Autodesk Inventor part; units mm, degrees
ref_plane "YZ Plane" through (0, 0, 0) normal (1, 0, 0) x (0, 1, 0)
ref_plane "XZ Plane" through (0, 0, 0) normal (0, 1, 0) x (-1, 0, 0)
ref_plane "XY Plane" through (0, 0, 0) normal (0, 0, 1) x (1, 0, 0)
sketch "Sketch1" plane through (0, 0, 0) normal (1, 0, 0) x (0, 1, 0)
  circle A0 centre (-9.1612, 46.1081) radius 0.5 construction
  circle A1 centre (-9.1612, 46.1081) radius 0.9 construction
  line L0 (0, 43.0329) -> (-28.9151, 45.5627) construction
  line L1 (1.0918, 43.1767) -> (-27.4928, 38.1364) construction
  line L2 (-1.0918, 51.3262) -> (-28.367, 41.3989) construction
  line L3 (0, 51.4699) -> (-28.9151, 48.9402) construction
  line L4 (17.609, 51.9698) -> (-38.9081, 36.826) construction
  line L5 (18.2302, 47.2514) -> (-40.2807, 47.2514) construction
  line L6 (-2.4562, 42.2517) -> (-3.9425, 12.3724) construction
  line L7 (-19.1091, 33.3894) -> (19.1091, 33.3894) construction
  line L8 (-15.9499, 49.3393) -> (15.9499, 17.4395) construction
  line L9 (-15.9953, 17.3941) -> (15.9953, 49.3847) construction
  line L10 (2.4672, 42.2517) -> (3.9506, 12.3724) construction
  line L11 (-4.2099, 47.2514) -> (-6.25, 6.2414) construction
  line L12 (4.2215, 47.2514) -> (6.2448, 6.4952) construction
  circle A2 centre (-12.7187, 42.5506) radius 0.9 construction
  line L13 (-11.8457, 45.2351) -> (-10.9619, 46.119) construction
  line L14 (-10.9619, 46.119) -> (-9.1941, 44.3513) construction
  line L15 (-12.7296, 44.3513) -> (-13.501, 42.9956) construction
  line L16 (-11.8457, 45.2351) -> (-12.7296, 44.3513) construction
  line L17 (-10.9619, 42.5835) -> (-12.2433, 41.7864) construction
  line L18 (-12.7296, 44.3513) -> (-10.9619, 42.5835) construction
  line L19 (-10.9619, 46.119) -> (-9.6062, 46.8904) construction
  line L20 (-9.1941, 44.3513) -> (-10.078, 43.4674) construction
  line L21 (-10.9619, 42.5835) -> (-10.078, 43.4674) construction
  circle A3 centre (-12.7187, 42.5506) radius 0.5 construction
  line L22 (-13.4028, 41.8664) -> (-9.1612, 46.1081) construction
  line L23 (-9.1941, 44.3513) -> (-8.3969, 45.6327) construction
  line L24 (0.0006, 41.0008) -> (0, 41.0008) construction
  line L25 (0.0006, 41.0001) -> (0, 41.0001) construction
  line L26 (-2.4567, 42.2414) -> (2.4677, 42.2414) construction
  line L27 (2.4672, 42.2517) -> (-2.4562, 42.2517) construction
  line L28 (3, 47.2514) -> (4.2185, 47.2514) construction
  line L29 (0, 48.3894) -> (0, 48.3894) construction
  line L30 (-4.2185, 47.2514) -> (-4.2099, 47.2514) construction
  line L31 (0, 51.4699) -> (0, 43.0329) construction
  line L32 (-1.0918, 51.3262) -> (1.0918, 43.1767) construction
  ellipse E0 centre (0, 47.2514) end of major axis (-3, 47.2514) minor radius 3 (0.0225, 44.2515) -> (-0.0225, 44.2515) ccw construction
  circle A4 centre (0, 47.2514) radius 3 construction
  ellipse E1 centre (0, 47.2514) end of major axis (4.2185, 47.2514) minor radius 4.2127 (4.2185, 47.2514) -> (-4.2185, 47.2514) ccw construction
  circle A5 centre (0, 47.2514) radius 4.2185 construction
  line L33 (-6.0016, 11.2344) -> (6.0096, 11.2344) construction
  line L34 (-3.9425, 12.3724) -> (3.9506, 12.3724) construction
  ellipse E2 centre (0, 6.2414) end of major axis (-5, 6.2414) minor radius 5 construction
  ellipse E3 centre (0, 6.2414) end of major axis (6.25, 6.2414) minor radius 6.2414 (-6.2423, 6.5518) -> (6.2393, 6.6057) ccw construction
  line L35 (-28.1887, 40.7336) -> (-33.0183, 39.4395) construction
  line L36 (-34.1303, 30.7554) -> (-31, 33.8856) construction
  line L37 (-42.8892, 48.6033) -> (-22.6298, 28.3438) construction
  circle A6 centre (-31.7936, 38.7324) radius 0.2 construction
  circle A7 centre (-33.0183, 39.4395) radius 0.2 construction
  circle A8 centre (-32.7595, 38.4736) radius 0.6398 construction
  circle A9 centre (-32.7595, 38.4736) radius 0.6398 construction
  line L38 (-33.6434, 39.3574) -> (-31.8756, 37.5897) construction
  line L39 (-33.6434, 39.3574) -> (-31.5728, 39.3574) construction
  line L40 (-27.4928, 38.1364) -> (-28.367, 41.3989) construction
  line L41 (-28.9151, 45.5627) -> (-28.9151, 48.9402) construction
  line L42 (-34.0028, 47.2514) -> (-25.2783, 38.5269) construction
  line L43 (-28.1887, 40.7336) -> (-22.3931, 42.2865) construction
  line L44 (-21.5614, 39.1823) -> (-22.7073, 43.4588) construction
  line L45 (-27.6711, 38.8017) -> (-21.8755, 40.3546) construction
  line L46 (-32.5007, 37.5076) -> (-27.6711, 38.8017) construction
  line L47 (-42.7094, 48.4234) -> (-41.2248, 46.9389) construction
  line L48 (-33.0183, 39.4395) -> (-32.5007, 37.5076) construction
  circle A10 centre (-32.5007, 37.5076) radius 0.2 construction
  circle A11 centre (-32.7595, 38.4736) radius 1.01 construction
  circle A12 centre (-33.7254, 38.2147) radius 0.2 construction
  circle A13 centre (-32.7595, 38.4736) radius 1.25 construction
  line L49 (-31.8756, 37.5897) -> (-33.2898, 36.1755) construction
  line L50 (-31.8756, 37.5897) -> (-32.9109, 35.7965) construction
  line L51 (-35.0576, 37.9432) -> (-33.6434, 39.3574) construction
  line L52 (-32.9109, 35.7965) -> (-33.8666, 34.8408) construction
  line L53 (-33.2898, 36.1755) -> (-35.0576, 37.9432) construction
  line L54 (-35.4365, 38.3222) -> (-32.9109, 35.7965) construction
  line L55 (-36.3923, 37.3664) -> (-35.4365, 38.3222) construction
  line L56 (-33.8666, 34.8408) -> (-36.3923, 37.3664) construction
  line L57 (-31, 33.8856) -> (-41.6066, 44.4922) construction
  line L58 (-44.7369, 41.362) -> (-34.1303, 30.7554) construction
  line L59 (-43.1717, 42.9271) -> (-32.5651, 32.3205) construction
  line L60 (-33.6434, 39.3574) -> (-35.4365, 38.3222) construction
  circle A14 centre (-46.5116, 43.1367) radius 1.0497 construction
  line L61 (-47.1835, 40.9802) -> (-44.2042, 43.9595) construction
  line L62 (-46.1769, 46.993) -> (-47.2764, 45.8935) construction
  line L63 (-43.7409, 42.358) -> (-42.6414, 43.4574) construction
  line L64 (-43.1717, 42.9271) -> (-45.2366, 44.992) construction
  line L65 (-47.2764, 45.8935) -> (-43.7409, 42.358) construction
  line L66 (-45.8947, 42.269) -> (-42.5137, 45.6501) construction
  line L67 (-41.6066, 44.4922) -> (-44.7369, 41.362) construction
  line L68 (-48.6681, 42.4647) -> (-42.7094, 48.4234) construction
  line L69 (-41.9671, 47.6812) -> (-47.9258, 41.7225) construction
  line L70 (-41.2248, 46.9389) -> (-47.1835, 40.9802) construction
  line L71 (-42.6414, 43.4574) -> (-46.1769, 46.993) construction
  line L72 (-44.1236, 47.0092) -> (-42.6391, 45.5247) construction
  line L73 (-41.2248, 46.9389) -> (-44.2042, 43.9595) construction
  circle A15 centre (-43.3813, 46.2669) radius 1.0497 construction
  line L74 (-47.1835, 40.9802) -> (-48.6681, 42.4647) construction
  line L75 (-47.2538, 43.8789) -> (-45.7693, 42.3944) construction
  circle A16 centre (-43.3813, 46.2669) radius 1.0497 construction
  circle A17 centre (-46.5116, 43.1367) radius 1.05 construction
  circle A18 centre (-43.3813, 46.2669) radius 1.3 construction
  circle A19 centre (-46.5116, 43.1367) radius 1.3 construction
  line L76 (-41.9671, 47.6812) -> (-47.9258, 41.7225) construction
  line L77 (-47.9258, 41.7225) -> (-49.6936, 43.4902) construction
  line L78 (-49.6936, 43.4902) -> (-43.7349, 49.4489) construction
  line L79 (-43.7349, 49.4489) -> (-41.9671, 47.6812) construction
  line L80 (-41.9671, 47.6812) -> (-42.0968, 46.0669) construction
  line L81 (-47.9258, 41.7225) -> (-46.3116, 41.8522) construction
  line L82 (-44.9465, 44.7018) -> (-45.2271, 42.9367) construction
  line L83 (-44.9465, 44.7018) -> (-43.1813, 44.9824) construction
  line L84 (-44.801, 45.617) -> (-44.0639, 44.8421) construction
  line L85 (-44.0639, 44.8421) -> (-45.1697, 43.7902) construction
  line L86 (-45.1697, 43.7902) -> (-45.9068, 44.5651) construction
  line L87 (-45.9068, 44.5651) -> (-44.801, 45.617) construction
  line L88 (-44.801, 48.3828) -> (-49.0061, 44.1777) construction
  line L89 (-49.0061, 44.1777) -> (-52.5417, 47.7132) construction
  line L90 (-52.5417, 47.7132) -> (-48.3365, 51.9184) construction
  line L91 (-48.3365, 51.9184) -> (-44.801, 48.3828) construction
  line L92 (-46.9035, 50.4854) -> (-51.1087, 46.2803) construction
  line L93 (-44.801, 48.3828) -> (-43.7755, 47.3573)
  line L94 (-43.7755, 47.3573) -> (-47.9806, 43.1522)
  line L95 (-47.9806, 43.1522) -> (-49.0061, 44.1777)
  line L96 (-49.0061, 44.1777) -> (-44.801, 48.3828)
  line L97 (-46.1769, 46.993) -> (-45.1584, 45.9744)
  line L98 (-45.1584, 45.9744) -> (-46.2578, 44.875)
  line L99 (-46.2578, 44.875) -> (-47.2764, 45.8935)
  line L100 (-47.2764, 45.8935) -> (-46.1769, 46.993)
  point P0 (0, 0)
  point P1 (0, 0)
  point P2 (0, 33.3894)
  point P3 (-6.009, 41)
  point P4 (0, 47.2514)
  point P5 (0, 47.2514)
  point P6 (0, 0)
  point P7 (0, 0)
  point P8 (0, 12.3724)
  point P9 (0, 0)
  point P10 (28.7519, 36.3712)
  point P11 (-45.0774, 43.878)
  dimension "d12" = 3
  dimension "d13" = 5
  dimension "d14" = 6.2414
  dimension "d4" = 41.01
  dimension "d5" = 6.2414
  dimension "d6" = 4.993
  dimension "d7" = 5.69
  dimension "d8" = 29.869
  dimension "d9" = 1.138
  dimension "d10" = 2
  dimension "d11" = 90
  dimension "d15" = 15
  dimension "d16" = 2.5
  dimension "d17" = 1.25
  dimension "d18" = 60
  dimension "d19" = 2
  dimension "d20" = 1
  dimension "d21" = 6
  dimension "d22" = 1
  dimension "d23" = 1.8
  dimension "d24" = 5
  dimension "d25" = 2
  dimension "d26" = 2.02
  dimension "d27" = 2.5
  dimension "d28" = 0.4
  dimension "d29" = 360
  dimension "d30" = 150
  dimension "d31" = 15
  dimension "d32" = 15
  dimension "d33" = 5
  dimension "d34" = 0.75
  dimension "d35" = 4.2134
  dimension "d36" = 2
  dimension "d37" = 2.1
  dimension "d38" = 2.6
  dimension "d39" = 2.6
  dimension "d40" = 2.5
  dimension "d41" = 5
  dimension "d42" = 5.947
extrude "Extrusion1" add sketch "Sketch1" along normal mid plane 8
sketch "Sketch2" plane through (-4, -49.0061, 44.1777) normal (0, -0.7071068, 0.7071068) x (1, 0, 0)
  line L0 (0, 0) -> (8, 0)
  line L1 (8, 5.947) -> (8, 0)
  line L2 (8, 5.947) -> (0, 5.947)
  line L3 (0, 0) -> (0, 5.947)
  line L4 (0, 0) -> (8, 5.947)
  line L5 (0, 5.947) -> (0, 0)
  line L6 (0, 5.947) -> (8, 0)
  line L7 (0, 5.947) -> (8, 5.947)
  line L8 (4, 5.947) -> (4, -0.1076) construction
  line L9 (0, 2.9735) -> (8, 3) construction
  circle A0 centre (0.75, 0.75) radius 0.75
  circle A1 centre (4, 2.9735) radius 1.8
  line L10 (0.1438, 1.1916) -> (0.9981, 0.0422)
  circle A2 centre (0.7353, 5.2019) radius 0.75
  line L11 (0.1319, 4.7563) -> (0.9787, 5.9113)
  circle A3 centre (7.25, 0.75) radius 0.75
  line L12 (7.8562, 1.1916) -> (7.0019, 0.0422)
  line L13 (7.8681, 4.7563) -> (7.0213, 5.9113)
  circle A4 centre (7.2647, 5.2019) radius 0.75
  line L14 (2.6994, 4.2179) -> (0.1438, 1.1916)
  line L15 (0.8749, 0) -> (4.5834, 1.2707)
  line L16 (7.1253, 5.947) -> (3.4953, 4.7013)
  line L17 (7.8681, 4.7563) -> (5.295, 1.7233)
  line L18 (0, 5.947) -> (8, 5.947)
  line L19 (8, 5.947) -> (8, 0)
  line L20 (8, 0) -> (0, 0)
  line L21 (0, 0) -> (0, 5.947)
  circle A5 centre (4, 2.9735) radius 0.8
  circle A6 centre (0.75, 0.75) radius 0.5
  circle A7 centre (7.2647, 5.2019) radius 0.5
  point P0 (4, 3.4142)
  point P1 (8, 5.3499)
  point P2 (7.3505, 5.947)
  point P3 (8, 5.0539)
  point P4 (7.8027, 4.6793)
  point P5 (5.4446, 1.8996)
  point P6 (0, 0.75)
  point P7 (0.2132, 1.2737)
  point P8 (2.5554, 4.0474)
  point P9 (7.1253, 5.947)
  point P10 (0.75, 0)
  point P11 (4, 3)
  dimension "d45" = 1.5
  dimension "d46" = 3.6
  dimension "d49" = 1.6
  dimension "d52" = 1
  dimension "d53" = 1
extrude "Extrusion2" cut sketch "Sketch2" against normal through all contours L4 A0 L0 | L3 A0 L4 | L3 A2 L6 L14 A0 | L15 A1 L6 A3 L0 | L3 A2 L6 L11 | A3 L6 L0 | A3 L12 L6 | L3 L6 A2 | L11 L6 A2 | L6 A2 L2 L16 A1 | L6 A3 L1 | A3 L6 L12 | L6 L12 A3 | L2 A2 L6 | A2 L2 L11 L6 | L6 L11 A2 | A3 L6 L17 A4 L1 | A3 L12 L6 | A4 L4 L1 | L4 A4 L2
extrude "Extrusion3" cut sketch "Sketch2" against normal through all contours A5 L4 L6 | L6 L4 A5 | L4 L6 A5 | L4 A5 L6
extrude "Extrusion4" cut sketch "Sketch2" against normal through all contours A6 L10 L4 | L4 L10 A6 | A6 L4 L10 | L4 A6 L10 | A7 L4 L13 | L13 L4 A7 | A7 L4 L13 | L13 L4 A7
properties part number "clamp_mechanism" material "Steel, Mild"
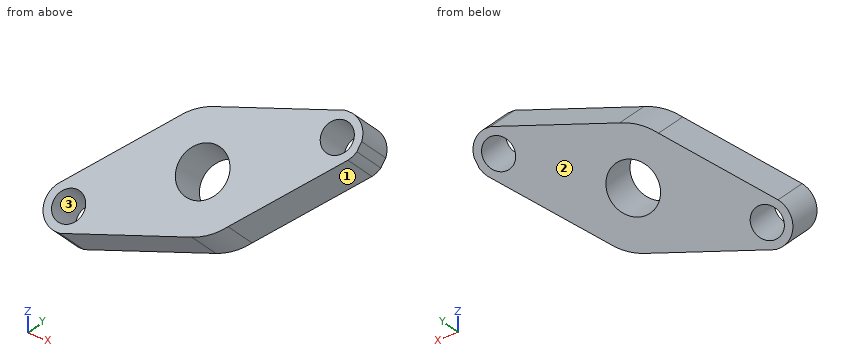
Design review of the part built by this model. Coordinates are the model's own, in mm. Face numbers are marked on the shaded views. Round coordinates to 2 decimals unless told otherwise and drop trailing zeros. Write each loop counter-clockwise with the first axis right and the second up, starting at its lowest first coordinate (ties: lowest second). Pieces come first, ordered by that corner, then holes.
Item 1: We need section A-A on x = 2.5. Write out the cut boundary in (y, z).
Item 2: Clearance check with flat-ended pins moving along their axes: pin 1 Ø1.5 at (y, z) = (-47.5, 45) entering from +X; pin 2 Ø1.5 at (x, z) = (-1, 44.5) entering from +Y; pin 3 Ø2 at (y, z) = (-46.5, 46) entering from -X. State where each tip first meets the part, or that it passes through.
Item 3: For probe 1 along X at (y, z) = (-45.8, 46.1); probe 2 along X at (y, z) = (-44.8, 47.25); probe 3 along Z at (x, y) = (1.5, -45.1), list the stretches that pass through material, from the lowest coordinate up.
Item 4: We need section B-B on x = 1.25. Write out the cut boundary in (y, z).
Item 5: The part is to be moulded in two halves that separate along Y. For the marked faces 1, 2 and 3, say which applies: +Y half, -Y half, draft (parallel to the pull), parting line (faces both ways), or undercut.
Returned:
1. outline: (-46.78, 46.4) - (-45.76, 45.38) - (-43.93, 47.21) - (-44.95, 48.23) - close
2. pin 1: stops at x = 1.87
2. pin 2: stops at y = -45.88
2. pin 3: stops at x = -3.12
3. probe 1: x = -1.8 to -0.46, 0.46 to 2.91
3. probe 2: x = 0.79 to 2.77, 3.76 to 4
3. probe 3: z = 46.03 to 47.89
4. outline: (-47.82, 45.36) - (-46.79, 44.34) - (-44.23, 46.9) - (-45.26, 47.93) - close
5. face 1: -Y half
5. face 2: +Y half
5. face 3: undercut
